Geometry: final body of the model. Coordinates: model frame, mm. A direction names the side the tool comes from. Round coordinates to 2 decimals unless told otherwise and drop trailing zeros. Write each loop counter-clockwise with the first axis right and the second up, starting at its lowest first coordinate (ties: lowest second). Pieces come first, ordered by that corner, then holes. Notation, with made-up numbers: M 33,-9.75 L 64,-9.75 A11 cw 64,-5.75 Z; hole C 45.25,84.5 d8. An arc over 180 degrees is marked long. Answer as CSV lines item,"result". Start each with the question number.
Q1. Ray query, probe 1 along X at (y, z) = (1.25, 1.9); probe 2 along X at (y, z) = (1.5, 1.85); probe 3 along Y at (x, z) = (4.25, 2.85). Return the intervals inside material, ascending.
Q2. Section query A-A on z = 1.2. Output: boundary loops of the cut face in (x, y).
Q3. Section query B-B on y = 1. Output: boundary loops of the cut face in (x, z).
Q4. Reachability of faces 1 (the flat face through (3, 11, 1)), 2 (the flat face through (-4.5, -13, 1)), 3 (the flat face through (-6, -14, 1)) from +Z, -Z, +X, -X, +Y, -Y: full face, straight path, thin tool, end or side. Return the list, or none.
Q5. First-contact query: pin 1 (1.5 mm diameter, centred on x = 3.5, z = 1.5, fed in from -Y). Flat tip, straight axial feed; report the tip coordinate or a pass-through.
Q6. Section query C-C on x = -4. Output: boundary loops of the cut face in (y, z), and give its area (3 significant figures).
Q7. Mould query, pull axis X, two halves, no side actions, for faces 4 (the flat face through (7.5, 0, 1)), 5 (the flat face through (6, -14, 1)), 6 (the flat face through (-3, 11, 1)). Classes: pulls with the +X half, pulls with the -X half, needs draft (parallel to the pull), parting line crosses it, or undercut.
Q8. Section query D-D on x = -2. Output: boundary loops of the cut face in (y, z).
```python
from build123d import *

# Parameters (mm, degrees)
SKETCH1_R           = 1
BOSS_EXTRUDE2_DEPTH = 3


with BuildPart() as part:
    # Sketch1 → Boss-Extrude2 (new body)
    with BuildSketch(Plane.XY):
        Polygon((-7.5, -14), (-4.5, -14), (-4.5, -11), (-1.5, -11), (-1.5, -14), (1.5, -14), (1.5, -11), (4.5, -11), (4.5, -14), (7.5, -14), (7.5, 14), (4.5, 14), (4.5, 11), (1.5, 11), (1.5, 14), (-1.5, 14), (-1.5, 11), (-4.5, 11), (-4.5, 14), (-7.5, 14), align=None)
        with Locations((-4.5, 1)):
            Circle(SKETCH1_R, mode=Mode.SUBTRACT)
        with Locations(Location((4.5, 1, 0), (0, 0, 180))):
            Circle(SKETCH1_R, mode=Mode.SUBTRACT)
    extrude(amount=BOSS_EXTRUDE2_DEPTH)


solid = part.part
```
Entries:
1,probe 1,"x = -7.5 to -5.47, -3.53 to 3.53, 5.47 to 7.5"
1,probe 2,"x = -7.5 to -5.37, -3.63 to 3.63, 5.37 to 7.5"
1,probe 3,"y = -11 to 0.03, 1.97 to 11"
2,outline,"M -7.5,-14 L -4.5,-14 L -4.5,-11 L -1.5,-11 L -1.5,-14 L 1.5,-14 L 1.5,-11 L 4.5,-11 L 4.5,-14 L 7.5,-14 L 7.5,14 L 4.5,14 L 4.5,11 L 1.5,11 L 1.5,14 L -1.5,14 L -1.5,11 L -4.5,11 L -4.5,14 L -7.5,14 Z; hole C -4.5,1 d2; hole C 4.5,1 d2"
3,outline,"M -7.5,0 L -5.5,0 L -5.5,3 L -7.5,3 Z; M -3.5,0 L 3.5,0 L 3.5,3 L -3.5,3 Z; M 5.5,0 L 7.5,0 L 7.5,3 L 5.5,3 Z"
4,face 1,"+Z, -Z, +Y"
4,face 2,"+Z, -Z, -Y"
4,face 3,"+Z, -Z, +X, -X, -Y"
5,pin 1,"stops at y = -11"
6,outline,"M -11,0 L 0.13,0 L 0.13,3 L -11,3 Z; M 1.87,0 L 11,0 L 11,3 L 1.87,3 Z"
6,area,"60.8 mm^2"
7,face 4,"pulls with the +X half"
7,face 5,"needs draft"
7,face 6,"undercut"
8,outline,"M -11,0 L 11,0 L 11,3 L -11,3 Z"
